The model under review builds one solid part; all positions refer to its coordinate system, in mm. A direction names the side the tool comes from. Round coordinates to 2 decimals unless told otherwise and drop trailing zeros. Order: outer loops, then holes, each group sorted by start corner. A loop starts at its lowest first (then second) coordinate and runs counter-clockwise, first axis right, second up. Notation, with made-up numbers: M 81.25,4.5 L 104.25,4.5 A26 ccw 104.25,26.5 Z; hole C 45.25,68.25 d2. An arc over 180 degrees is marked long. Answer as a JSON object with one key per item and string values. Group by question number.
1) Consider section D-D, the plane z = -30. Write out the cut boundary in (x, y), then the cut area to 3 significant figures.
2) To check wall thickness, follow line 1 (Z direction, x = 40.5, y = 11.5); line 2 (X direction, y = 10.75, z = -36.5); line 3 (X direction, y = 11, z = -17.5). State the ranges of each line that lie inside material, in increasing order.
3) Consider section C-C, the plane z = -25.5. Write out the cut boundary in (x, y), then the cut area to 3 significant figures.
4) Consider section A-A, the plane x = 28.5. Write out the cut boundary in (y, z).
5) The part is to be moulded in two halves that separate along Z. For faces 6 (the flat face through (38.7, 3, -3.5)), 7 (the flat face through (24, 0, -21)), 8 (the cylindrical face through (1.711, 7.395, -41.196)), 9 (the flat face through (24, 6, -3)), say which applies: +Z half, -Z half, draft (parallel to the pull), parting line (faces both ways), or undercut.
6) For faces 1 (the cylindrical face through (42.452, 10.437, -36.934)), 2 (the cylindrical face through (6.6, 9.1, -27.4)), 3 (the flat face through (23, 7, -2)), 4 (the cylindrical face through (26.354, 9.676, -41.521)), 5 (the flat face through (3, 3, -37)), list the 3-axis set-ups (+Z, -Z, +X, -X, +Y, -Y) from which the entire face can be reached by the end or side of a thin tool; tool diameter is ignored.
7) Insertion check: pin 1 Ø3.5 at (x, z) = (39.5, -37) entering from -Y; pin 2 Ø3.5 at (x, z) = (23.5, -1) entering from +Y; pin 3 Ø2.5 at (y, z) = (10.5, -1) entering from +X. Each pin has a flat end and moves straight along its axis. Give the tip position at first contact, or say it passes through.
8) Consider section B-B, the plane y = 13. Write out the cut boundary in (x, z), then the cut area to 3 significant figures.
Autodesk Inventor part; units mm, degrees
ref_plane "YZ Plane" through (0, 0, 0) normal (1, 0, 0) x (0, 1, 0)
ref_plane "XZ Plane" through (0, 0, 0) normal (0, 1, 0) x (-1, 0, 0)
ref_plane "XY Plane" through (0, 0, 0) normal (0, 0, 1) x (1, 0, 0)
sketch "Sketch1" plane through (0, 0, 0) normal (0, 1, 0) x (-1, 0, 0)
  line L0 (0, 0) -> (-47, 0)
  line L1 (-47, 0) -> (-47, -43)
  line L2 (-47, -43) -> (0, -43)
  line L3 (0, -43) -> (0, 0)
  line L4 (-13, -40) -> (-34, -40) construction
  line L5 (-34, -40) -> (-34, -3) construction
  line L6 (-34, -3) -> (-13, -3) construction
  line L7 (-13, -3) -> (-13, -40) construction
  point P0 (-23.5, -40)
  point P1 (-23.5, -43)
  point P2 (-13, -21.5)
  point P3 (0, -21.5)
  dimension "d2" = 21
  dimension "d3" = 37
  dimension "d11" = 13
  dimension "d12" = 3
extrude "Extrusion1" add sketch "Sketch1" along normal blind 3
sketch "Sketch2" plane through (0, 3, 0) normal (0, 1, 0) x (1, 0, 0)
  line L0 (0, 0) -> (47, 0)
  line L1 (47, 0) -> (47, 43)
  line L2 (47, 43) -> (0, 43)
  line L3 (0, 43) -> (0, 0)
  line L4 (13, 40) -> (34, 40)
  line L5 (34, 40) -> (34, 3)
  line L6 (34, 3) -> (13, 3)
  line L7 (13, 3) -> (13, 40)
  point P0 (13, 21.5)
  point P1 (0, 21.5)
  point P2 (23.5, 40)
  point P3 (23.5, 43)
  dimension "d15" = 37
  dimension "d16" = 21
extrude "Extrusion2" add sketch "Sketch2" along normal blind 12
sketch "Sketch4" plane through (0, 15, 0) normal (0, 1, 0) x (1, 0, 0)
  line L0 (34, 3) -> (13, 3)
  line L1 (0, 0) -> (47, 0)
  line L2 (26, 3) -> (21, 3)
  line L3 (21, 3) -> (21, 0)
  line L4 (21, 0) -> (26, 0)
  line L5 (26, 0) -> (26, 3)
  point P0 (23.5, 3)
  point P1 (23.5, 3)
  dimension "d19" = 5
extrude "Extrusion3" cut sketch "Sketch4" against normal blind 8
sketch "Sketch5" plane through (0, 15, 0) normal (0, 1, 0) x (1, 0, 0)
  line L0 (47, 43) -> (0, 43)
  line L1 (0, 43) -> (0, 0)
  line L2 (6.5, 36.5) -> (40.5, 36.5) construction
  line L3 (40.5, 36.5) -> (40.5, 6.5) construction
  line L4 (40.5, 6.5) -> (6.5, 6.5) construction
  line L5 (6.5, 6.5) -> (6.5, 36.5) construction
  point P0 (6.5, 21.5)
  point P1 (0, 21.5)
  point P2 (23.5, 36.5)
  point P3 (23.5, 43)
  dimension "d22" = 6.5
  dimension "d23" = 6.5
hole "Hole1" at (6.5, 15, -36.5) at (6.5, 15, -6.5) at (40.5, 15, -6.5) at (40.5, 15, -36.5) direction (0, -1, 0) diameter 4 end through all
sketch "Sketch7" plane through (47, 0, 0) normal (1, 0, 0) x (0, 0, -1)
  line L0 (0, 0) -> (0, 15)
  circle A0 centre (21.6469, 9) radius 2.25
  circle A1 centre (29.6469, 9) radius 2.25
  circle A2 centre (13.6469, 9) radius 2.25
  dimension "d42" = 4.5
  dimension "d43" = 8
  dimension "d44" = 8
  dimension "d54" = 15
  dimension "d55" = 9
extrude "Extrusion5" cut sketch "Sketch7" against normal through all
sketch "Sketch8" plane through (47, 0, -43) normal (0, 0, -1) x (-1, 0, 0)
  line L0 (0, 0) -> (47, 0)
  line L1 (0, 15) -> (47, 15)
  line L2 (23.5, 15) -> (23.5, 0) construction
  circle A0 centre (18.5, 9) radius 2.25
  circle A1 centre (28.5, 9) radius 2.25
  dimension "d47" = 4.5
  dimension "d48" = 4.5
  dimension "d49" = 5
  dimension "d50" = 5
  dimension "d56" = 15
  dimension "d57" = 9
extrude "Extrusion6" cut sketch "Sketch8" against normal up to next
fillet "Fillet2" radius 6 4 edges at (0, 7.5, 0) (47, 7.5, 0) (47, 7.5, -43) (0, 7.5, -43)
sketch "Sketch9" plane through (0, 0, 0) normal (0, -1, 0) x (1, 0, 0)
  circle A0 centre (40.5, -6.5) radius 2
  circle A1 centre (6.5, -36.5) radius 2
  circle A2 centre (6.5, -6.5) radius 2
  circle A3 centre (40.5, -36.5) radius 2
  line L0 (6.5, -10.5415) -> (3, -8.5207)
  line L1 (3, -8.5207) -> (3, -4.4793)
  line L2 (3, -4.4793) -> (6.5, -2.4585)
  line L3 (6.5, -2.4585) -> (10, -4.4793)
  line L4 (10, -4.4793) -> (10, -8.5207)
  line L5 (10, -8.5207) -> (6.5, -10.5415)
  line L6 (10, -38.5207) -> (6.5, -40.5415)
  line L7 (6.5, -40.5415) -> (3, -38.5207)
  line L8 (3, -38.5207) -> (3, -34.4793)
  line L9 (3, -34.4793) -> (6.5, -32.4585)
  line L10 (6.5, -32.4585) -> (10, -34.4793)
  line L11 (10, -34.4793) -> (10, -38.5207)
  line L12 (37, -38.5207) -> (37, -34.4793)
  line L13 (37, -34.4793) -> (40.5, -32.4585)
  line L14 (40.5, -32.4585) -> (44, -34.4793)
  line L15 (44, -34.4793) -> (44, -38.5207)
  line L16 (44, -38.5207) -> (40.5, -40.5415)
  line L17 (40.5, -40.5415) -> (37, -38.5207)
  line L18 (37, -8.5207) -> (37, -4.4793)
  line L19 (37, -4.4793) -> (40.5, -2.4585)
  line L20 (40.5, -2.4585) -> (44, -4.4793)
  line L21 (44, -4.4793) -> (44, -8.5207)
  line L22 (44, -8.5207) -> (40.5, -10.5415)
  line L23 (40.5, -10.5415) -> (37, -8.5207)
  point P0 (0, 0)
  dimension "d58" = 7
extrude "Extrusion7" cut sketch "Sketch9" against normal blind 6
equation "\"d23\" = d22"
equation "\"d44\" = d43"
equation "\"d48\" = d47"
equation "\"d50\" = d49"
properties part number "dht22_case_bottom"
Results list:
{
 "1": {"outline": "M 0,0 L 47,0 L 47,6.78 L 34,6.78 L 34,3 L 13,3 L 13,6.78 L 0,6.78 Z; M 0,11.22 L 13,11.22 L 13,15 L 0,15 Z; M 34,11.22 L 47,11.22 L 47,15 L 34,15 Z", "area": "337 mm^2"},
 "2": {"line 1": "-43 to -38.5, -34.5 to -8.5, -4.5 to 0", "line 2": "0 to 4.5, 8.5 to 13, 34 to 38.5, 42.5 to 47", "line 3": "0 to 13, 34 to 47"},
 "3": {"outline": "M 0,0 L 47,0 L 47,15 L 34,15 L 34,3 L 13,3 L 13,15 L 0,15 Z", "area": "453 mm^2"},
 "4": {"outline": "M 0,-43 L 6.75,-43 L 6.75,-40 L 3,-40 L 3,-3 L 15,-3 L 15,0 L 0,0 Z; M 11.25,-43 L 15,-43 L 15,-40 L 11.25,-40 Z"},
 "5": {"face 6": "undercut", "face 7": "draft", "face 8": "-Z half", "face 9": "undercut"},
 "6": {"face 1": "+Y, -Y", "face 2": "+X, -X", "face 3": "+Z, +Y", "face 4": "-Z", "face 5": "-Y"},
 "7": {"pin 1": "y = 6", "pin 2": "y = 7", "pin 3": "x = 45.68"},
 "8": {"outline": "M 0,-37 A6 ccw 6,-43 L 41,-43 A6 ccw 47,-37 L 47,-6 A6 ccw 41,0 L 26,0 L 26,-3 L 34,-3 L 34,-40 L 13,-40 L 13,-3 L 21,-3 L 21,0 L 6,0 A6 ccw 0,-6 Z; hole C 6.5,-36.5 d4; hole C 6.5,-6.5 d4; hole C 40.5,-36.5 d4; hole C 40.5,-6.5 d4", "area": "1,150 mm^2"}
}
